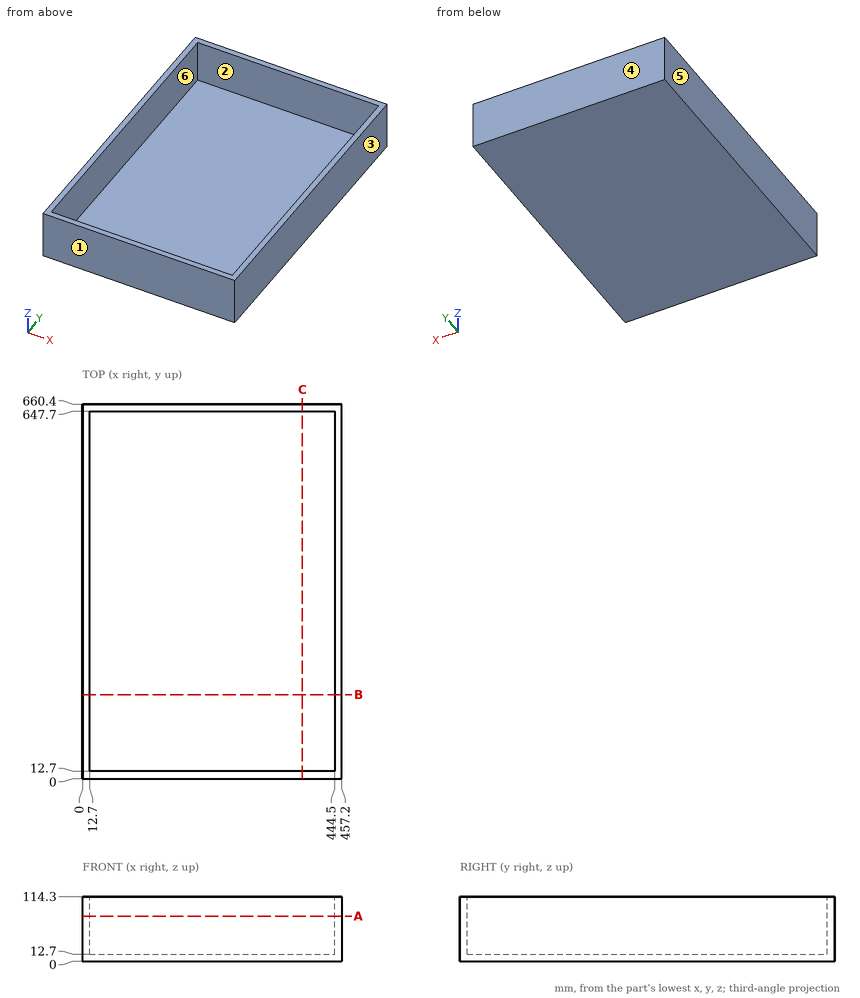
Print and shaded views of the part. All mm, measured from the part's lowest x, y and z. A direction names the side the tool comes from. Round coordinates to 2 decimals unless told otherwise and drop trailing zeros. Write each loop counter-clockwise with the first axis right and the second up, starting at its lowest first coordinate (ties: lowest second). Pieces come first, ordered by that corner, then holes.
(1) Mould opens along Y. For the marked faces 1, 2, 3 and 4 say: pulls with the +Y half, pulls with the -Y half, needs draft (parallel to the pull), parting line crosses it, or undercut.
(2) Slice it at A-A, the plane z = 80. Write the cut outline in (x, y), and give its area (3 significant figures).
(3) Probe line 1 along Y through (x, z) = (21, 77.5); line 2 along X through (y, z) = (158, 19.5); line 3 along Z through (x, y) = (274.5, 183). List the from-to ranges inside material, lowest first.
(4) Slice it at C-C, the plane x = 387.5. Write the cut outline in (y, z).
(5) Slice it at B-B, the plane y = 148. Write the cut outline in (x, z), and give its area (3 significant figures).
(6) 3-axis set-ups, long thin cutter, end or side, ignore diameter. For the marked faces 5 and 6: which of +Z, -Z, +X, -X, +Y, -Y reach the whole face in a straight line?
(7) Drop a flat-ended pin along its axis: P1, Ø6, axis at x = 111.5, y = 164.5, coming from the +Z side. Give the stop position or say it passes through.
From the geometry:
1. face 1: pulls with the -Y half
1. face 2: undercut
1. face 3: needs draft
1. face 4: pulls with the +Y half
2. outline: (0, 0) - (457.2, 0) - (457.2, 660.4) - (0, 660.4) - close; hole (12.7, 12.7) - (444.5, 12.7) - (444.5, 647.7) - (12.7, 647.7) - close
2. area: 27,700 mm2
3. line 1: y = 0 to 12.7, 647.7 to 660.4
3. line 2: x = 0 to 12.7, 444.5 to 457.2
3. line 3: z = 0 to 12.7
4. outline: (0, 0) - (660.4, 0) - (660.4, 114.3) - (647.7, 114.3) - (647.7, 12.7) - (12.7, 12.7) - (12.7, 114.3) - (0, 114.3) - close
5. outline: (0, 0) - (457.2, 0) - (457.2, 114.3) - (444.5, 114.3) - (444.5, 12.7) - (12.7, 12.7) - (12.7, 114.3) - (0, 114.3) - close
5. area: 8,390 mm2
6. face 5: +Z, -Z, -X, +Y, -Y
6. face 6: +Z
7. P1: stops at z = 12.7
